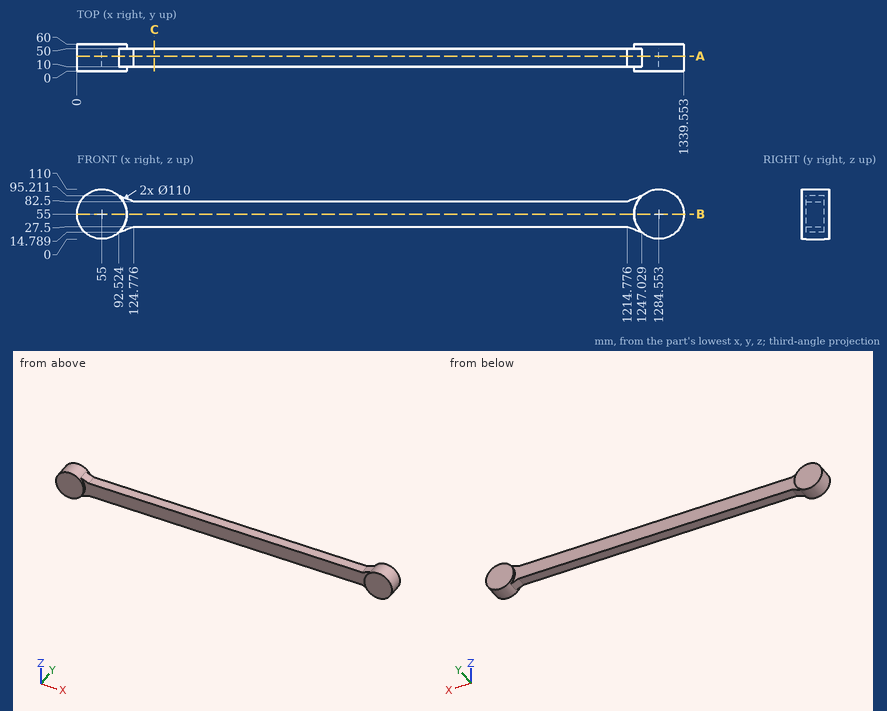
The drawing under review shows one solid part. Ordinate dimensions are in mm from its lowest x, y, z. Round coordinates to 2 decimals unless told otherwise and drop trailing zeros. Write each loop counter-clockwise with the first axis right and the second up, starting at its lowest first coordinate (ties: lowest second). Pieces come first, ordered by that corner, then holes. Notation, with made-up numbers: (33.5, 54) - (43.5, 54) arc R34 ccw to (43.5, 84) - close; hole circle Ø8 at (8.5, 81). An arc over 180 degrees is marked (long way). Use a Markdown table: item, result. Add a question column.
1. Clearance check with flat-ended pins moving along their axes: pin 1 (8 mm diameter, centred on y = 34, z = 34, fed in from -X); pin 2 (4 mm diameter, centred on x = 378.5, y = 33, fed in from +Z); pin 3 (2 mm diameter, centred on x = 425.5, z = 28.5, fed in from +Y). State where each tip first meets the part, or that it passes through.
2. We need section B-B (z = 55). State the section outline as (x, y) points.
3. Wall thickness on probe 1 along X at (y, z) = (56, 51.5) (1 decimal); probe 2 along Z at (x, y) = (912, 46); probe 3 along Y at (x, z) = (795, 46.5): over which ranges is each line inside the solid? List them lowest first.
4. We need section A-A (y = 33.5). State the section outline as (x, z) points (1 decimal), then the cut area to 3 significant figures.
5. We need section C-C (x = 171). State the section outline as (y, z) points, then the cut area to 3 significant figures.
Output:
| question | item | result |
|---|---|---|
| 1 | pin 1 | stops at x = 2.69 |
| 1 | pin 2 | stops at z = 82.5 |
| 1 | pin 3 | stops at y = 50 |
| 2 | outline | (0, 0) - (110, 0) - (110, 10) - (1229.55, 10) - (1229.55, 0) - (1339.55, 0) - (1339.55, 60) - (1229.55, 60) - (1229.55, 50) - (110, 50) - (110, 60) - (0, 60) - close |
| 3 | probe 1 | x = 0.1 to 109.9, 1229.7 to 1339.4 |
| 3 | probe 2 | z = 27.5 to 82.5 |
| 3 | probe 3 | y = 10 to 50 |
| 4 | outline | (92.5, 14.8) - (124.8, 27.5) - (1214.8, 27.5) - (1247, 14.8) arc R55 ccw (long way) to (1247, 95.2) - (1214.8, 82.5) - (124.8, 82.5) - (92.5, 95.2) arc R55 ccw (long way) to start |
| 4 | area | 81,400 mm2 |
| 5 | outline | (10, 27.5) - (50, 27.5) - (50, 82.5) - (10, 82.5) - close |
| 5 | area | 2,200 mm2 |
